```python
from build123d import *

# Parameters (mm, degrees)
SKETCH2_R           = 9
BOSS_EXTRUDE2_DEPTH = 10
SKETCH3_R           = 8
CUT_EXTRUDE1_DEPTH  = 5
SKETCH4_W           = 4.35
SKETCH4_H           = 6.15
CUT_EXTRUDE2_DEPTH  = 6


with BuildPart() as part:
    # Sketch2 → Boss-Extrude2 (new body)
    with BuildSketch(Plane(origin=(0, 0, 0), x_dir=(1, 0, 0), z_dir=(0, 1, 0))):
        Circle(SKETCH2_R)
    extrude(amount=BOSS_EXTRUDE2_DEPTH)

    # Sketch3 → Cut-Extrude1 (cut)
    with BuildSketch(Plane(origin=(0, 10, 0), x_dir=(1, 0, 0), z_dir=(0, 1, 0))):
        Circle(SKETCH3_R)
    extrude(amount=-CUT_EXTRUDE1_DEPTH, mode=Mode.SUBTRACT)

    # Sketch4 → Cut-Extrude2 (cut, through all)
    with BuildSketch(Plane(origin=(0, 5, 0), x_dir=(1, 0, 0), z_dir=(0, 1, 0))):
        with Locations((2.75, 0)):
            Rectangle(SKETCH4_W, SKETCH4_H)
        with Locations((-2.75, 0)):
            Rectangle(SKETCH4_W, SKETCH4_H)
    extrude(amount=-CUT_EXTRUDE2_DEPTH, mode=Mode.SUBTRACT)


solid = part.part
```
Can you work these out from the model? Positions are in its coordinate system, mm. A direction names the side the tool comes from. Round coordinates to 2 decimals unless told otherwise and drop trailing zeros. Loops run counter-clockwise (first coordinate to the right, second up) from the corner with the lowest first, then second, coordinate; pieces in that order, holes last. Notation, with made-up numbers: M 1.25,6 L 60.25,6 A18 ccw 60.25,29 Z; hole C 86,29.25 d7. An arc over 180 degrees is marked long. Write item = value, one per line. Start each with the question number.
(1) I'm going to push flat-ended pins straight in: P1, Ø6, axis at y = 7, z = 5.5, coming from the -X side; P2, Ø6, axis at y = 3.5, z = -7, coming from the -X side; P3, Ø1.3, axis at x = -3, y = 2, coming from the +Z side. Where does each tip first touch, or does it pass through?
(2) Suppose I cut it at B-B on x = 4.5. Write out the boundary of the cut face in (y, z) (3 decimals), plus the area to 3 significant figures.
(3) Suppose I cut it at A-A on y = 2. Write out the boundary of the cut face in (x, z) (3 decimals).
(4) Which directions (+Z, -Z, +X, -X, +Y, -Y) give clear straight access to the entire face, cutting with the end or side of a thin tool? Please do faces 4 (the face through (0, 5, 0)), 5 (the face through (-0.575, 3, 0)).
(5) Suppose I cut it at C-C on z = 0. Write out the boundary of the cut face in (x, y) (3 decimals).
(6) Suppose I cut it at D-D on x = 0. Write out the boundary of the cut face in (y, z).
(7) If we mould it in two halves opening along X, with no side actions, what happens to faces 1 (the face through (0, 0, 0)), 2 (the face through (-3, 3, -3.075)), 3 (the face through (-1.172, 4.93, -8.923))? For each: released by +X, released by -X, zero draft, split by the parting line, or undercut.
(8) I need wall thicknesses on line 1 along X through (y, z) = (8, 0); line 2 along Y through (x, z) = (-4, -4). Which ranges of each line are inside material? Lowest first, please.
Answer block:
q1.P1 = -8.65
q1.P2 = -8.06
q1.P3 = 8.69
q2.outline = M 0,-7.794 L 10,-7.794 L 10,-6.614 L 5,-6.614 L 5,-3.075 L 0,-3.075 Z; M 0,3.075 L 5,3.075 L 5,6.614 L 10,6.614 L 10,7.794 L 0,7.794 Z
q2.area = 59.0 mm²
q3.outline = C 0,0 d18; hole M -4.925,-3.075 L -0.575,-3.075 L -0.575,3.075 L -4.925,3.075 Z; hole M 0.575,-3.075 L 4.925,-3.075 L 4.925,3.075 L 0.575,3.075 Z
q4.face_4 = +Y
q4.face_5 = +Y, -Y
q5.outline = M -9,0 L -4.925,0 L -4.925,5 L -8,5 L -8,10 L -9,10 Z; M -0.575,0 L 0.575,0 L 0.575,5 L -0.575,5 Z; M 4.925,0 L 9,0 L 9,10 L 8,10 L 8,5 L 4.925,5 Z
q6.outline = M 0,-9 L 10,-9 L 10,-8 L 5,-8 L 5,8 L 10,8 L 10,9 L 0,9 Z
q7.face_1 = zero draft
q7.face_2 = undercut
q7.face_3 = split by the parting line
q8.line_1 = -9 to -8, 8 to 9
q8.line_2 = 0 to 5
